from build123d import *

# Parameters (mm, degrees)
F0_W      = 38.1
F0_H      = 82.55
F1_DEPTH  = 57.15
F3_DEPTH  = 48.006
F5_DEPTH  = 38.1
F6_R      = 5.08
F7_R      = 5.08
F8_R      = 5.08
F9_R      = 5.08
F10_R     = 5.08
F11_R     = 6.35
F12_DEPTH = 25.4


with BuildPart() as f1:
    # F0 (on Front) → F1 (new body)
    with BuildSketch(Plane.XZ):
        Rectangle(F0_W, F0_H)
    extrude(amount=F1_DEPTH)

    # F2 (on face) → F3 (cut)
    with BuildSketch(Plane.YZ.offset(19.05)):
        Polygon((-6.35, 34.925), (-57.15, 34.925), (-57.15, -41.275), (-50.8, -41.275), (-50.8, -34.925), (-6.35, -34.925), align=None)
    extrude(amount=-F3_DEPTH, mode=Mode.SUBTRACT)

    # F4 (on face) → F5 (join)
    with BuildSketch(Plane.YZ.offset(19.05)):
        Polygon((-50.8, -41.275), (-50.8, -34.925), (-85.9860533047, -10.6037642213), (-89.5966880699, -15.8273469566), align=None)
    extrude(amount=-F5_DEPTH)

    # F6
    f6_edges = [f1.edges().sort_by_distance(p)[0] for p in [
        (0, 0, 41.275),
    ]]
    fillet(f6_edges, radius=F6_R)

    # F7
    f7_edges = [f1.edges().sort_by_distance(p)[0] for p in [
        (0, -6.35, 34.925),
    ]]
    fillet(f7_edges, radius=F7_R)

    # F8
    f8_edges = [f1.edges().sort_by_distance(p)[0] for p in [
        (0, 0, -41.275),
    ]]
    fillet(f8_edges, radius=F8_R)

    # F9
    f9_edges = [f1.edges().sort_by_distance(p)[0] for p in [
        (0, -6.35, -34.925),
    ]]
    fillet(f9_edges, radius=F9_R)

    # F10
    f10_edges = [f1.edges().sort_by_distance(p)[0] for p in [
        (0, -50.8, -34.925),
        (0, -50.8, -41.275),
    ]]
    fillet(f10_edges, radius=F10_R)

    # F11 (on face) → F12 (cut)
    with BuildSketch(Plane.XY.offset(41.275)):
        with Locations((0, -38.1)):
            Circle(F11_R)
    extrude(amount=-F12_DEPTH, mode=Mode.SUBTRACT)


solid = f1.part
CAD build for the part. Positions are in the model's coordinates, mm. A direction names the side the tool comes from. Give positions to 0.01 mm unless a question says otherwise; leave off trailing zeros. Order: outer loops, then holes, each group sorted by start corner. A loop starts at its lowest first (then second) coordinate and runs counter-clockwise, first axis right, second up. Notation, with made-up numbers: (33.5, 74) - (56.5, 74) arc R19 ccw to (56.5, 88) - close; hole circle Ø9 at (29.25, -15). An arc over 180 degrees is marked (long way). Answer in a Markdown table with one row per item.
1. Probe probe 1 along X at (y, z) = (-38, 39); probe 2 along Z at (x, y) = (-7.5, -33.5) (3 decimals); probe 3 along Y at (x, z) = (-12.5, 21). List the from-to ranges inside material, lowest first. Write a range as [from, to].
Data:
| item | result |
|---|---|
| probe 1 | x = [-19.05, -6.35], [6.35, 19.05] |
| probe 2 | z = [-41.275, -34.925], [34.925, 41.275] |
| probe 3 | y = [-6.35, 0] |
2. Tool access for faces 5 (the flat face through (0, -57.15, 38)), 6 (the flat face through (0, -29, 34.925)), 7 (the cylindrical face through (-0.27, -50.71, -34.7)): list every direction of +Z, -Z, +X, -X, +Y, -Y with a clear straight run to the whole face (end or side of a thin tool).
Data:
| item | result |
|---|---|
| face 5 | +Z, +X, -X, -Y |
| face 6 | +X, -X, -Y |
| face 7 | +X, -X |
3. Pull direction Z, two halves, no side cores. Call faces 1 (the flat face through (0, -31, -34.925)), 2 (the flat face through (19.05, -5, -3)), 3 (the flat face through (0, -6.35, 0)), 4 (the flat face through (0.267, -87.766, -13.179)): pulls with the +Z half, pulls with the -Z half, needs draft (parallel to the pull), parting line crosses it, or undercut.
Data:
| item | result |
|---|---|
| face 1 | undercut |
| face 2 | needs draft |
| face 3 | undercut |
| face 4 | pulls with the +Z half |
4. Saw through at A-A, the plane y = -38.1. Give the cut face in (x, z) (3 decimals).
Data:
| item | result |
|---|---|
| outline | (-19.05, -41.275) - (19.05, -41.275) - (19.05, -34.925) - (-19.05, -34.925) - close; (-19.05, 34.925) - (-6.35, 34.925) - (-6.35, 41.275) - (-19.05, 41.275) - close; (6.35, 34.925) - (19.05, 34.925) - (19.05, 41.275) - (6.35, 41.275) - close |
5. Saw through at D-D, the plane x = 9. Give the cut face in (y, z) (3 decimals), plus the area to 3 significant figures.
Data:
| item | result |
|---|---|
| outline | (-89.597, -15.827) - (-52.069, -40.443) arc R5.08 ccw to (-49.283, -41.275) - (-5.08, -41.275) arc R5.08 ccw to (0, -36.195) - (0, 36.195) arc R5.08 ccw to (-5.08, 41.275) - (-57.15, 41.275) - (-57.15, 34.925) - (-11.43, 34.925) arc R5.08 cw to (-6.35, 29.845) - (-6.35, -29.845) arc R5.08 cw to (-11.43, -34.925) - (-49.215, -34.925) arc R5.08 cw to (-52.104, -34.024) - (-85.986, -10.604) - close |
| area | 1,390 mm² |
6. Saw through at B-B, the plane y = -13.5. Give the cut face in (x, z) (3 decimals).
Data:
| item | result |
|---|---|
| outline | (-19.05, -41.275) - (19.05, -41.275) - (19.05, -34.925) - (-19.05, -34.925) - close; (-19.05, 34.925) - (19.05, 34.925) - (19.05, 41.275) - (-19.05, 41.275) - close |
7. Saw through at C-C, the plane x = 0. Give the cut face in (y, z) (3 decimals), plus the area to 3 significant figures.
Data:
| item | result |
|---|---|
| outline | (-89.597, -15.827) - (-52.069, -40.443) arc R5.08 ccw to (-49.283, -41.275) - (-5.08, -41.275) arc R5.08 ccw to (0, -36.195) - (0, 36.195) arc R5.08 ccw to (-5.08, 41.275) - (-31.75, 41.275) - (-31.75, 34.925) - (-11.43, 34.925) arc R5.08 cw to (-6.35, 29.845) - (-6.35, -29.845) arc R5.08 cw to (-11.43, -34.925) - (-49.215, -34.925) arc R5.08 cw to (-52.104, -34.024) - (-85.986, -10.604) - close; (-57.15, 34.925) - (-44.45, 34.925) - (-44.45, 41.275) - (-57.15, 41.275) - close |
| area | 1,310 mm² |
8. Flat gauge pins, fed straight in: pin 1 (1 mm diameter, centred on x = 6.5, y = -72.5, fed in from +Z); pin 2 (4 mm diameter, centred on x = 9.5, z = -5.5, fed in from -Y); pin 3 (11.5 mm diameter, centred on x = 6, z = -8, fed in from -Y); pin 4 (12 mm diameter, centred on y = -33.5, z = -25.5, fed in from -X). Where does each tip first touch, or does it go through?
Data:
| item | result |
|---|---|
| pin 1 | stops at z = -19.58 |
| pin 2 | stops at y = -6.35 |
| pin 3 | stops at y = -88.16 |
| pin 4 | passes through |
